from build123d import *

# Parameters (mm, degrees)
F0_W     = 0.6
F0_H     = 1.6
F1_DEPTH = 5
F3_DEPTH = 5
F4_W     = 5
F4_H     = 5
F5_DEPTH = 25


with BuildPart() as f1:
    # F0 (on Top) → F1 (new body)
    with BuildSketch(Plane.XY):
        with BuildLine():
            ThreePointArc((50, 7.5), (48.535534, 11.035534), (45, 12.5))
            Line((45, 12.5), (-45, 12.5))
            ThreePointArc((-45, 12.5), (-48.535534, 11.035534), (-50, 7.5))
            Line((-50, 7.5), (-50, -7.5))
            ThreePointArc((-50, -7.5), (-48.535534, -11.035534), (-45, -12.5))
            Line((-45, -12.5), (45, -12.5))
            ThreePointArc((45, -12.5), (48.535534, -11.035534), (50, -7.5))
            Line((50, -7.5), (50, 7.5))
        make_face()
        with Locations((-41, 0)):
            Rectangle(F0_W, F0_H, mode=Mode.SUBTRACT)
        with Locations((-35, 0)):
            Rectangle(F0_W, F0_H, mode=Mode.SUBTRACT)
        with Locations((15, 0)):
            Rectangle(F0_W, F0_H, mode=Mode.SUBTRACT)
        with Locations((21, 0)):
            Rectangle(F0_W, F0_H, mode=Mode.SUBTRACT)
    extrude(amount=F1_DEPTH)

    # F2 (on face) → F3 (join)
    with BuildSketch(Plane.XY.offset(5)):
        Polygon((25, -10.15), (27, -10.15), (27, 10.15), (45.5, 10.15), (45.5, -10.15), (47.5, -10.15), (47.5, 10.15), (47.5, 11.65), (25, 11.65), (25, 10.15), align=None)
    extrude(amount=F3_DEPTH)

    # F4 (on face) → F5 (cut)
    with BuildSketch(Plane(origin=(0, 11.65, 0), x_dir=(-1, 0, 0), z_dir=(0, 1, 0))):
        with Locations((-43, 7.5)):
            Rectangle(F4_W, F4_H)
    extrude(amount=-F5_DEPTH, mode=Mode.SUBTRACT)


solid = f1.part
Could you check a few things on this model? Use its own coordinates, in mm. A direction names the side the tool comes from. Give positions to 0.01 mm unless a question says otherwise; leave off trailing zeros. Loops run counter-clockwise (first coordinate to the right, second up) from the corner with the lowest first, then second, coordinate; pieces in that order, holes last. Notation, with made-up numbers: (-15.5, 21) -> (10.5, 21) arc R14 ccw to (10.5, 47) -> close; hole circle Ø6 at (-27, -17). An arc over 180 degrees is marked (long way). Answer as CSV lines item,"result". Start each with the question number.
(1) If we section it at A-A on y = -4.25: Write out the boundary of the cut face in (x, z).
(2) If we section it at B-B on x = -2: Write out the boundary of the cut face in (y, z), then the cut area to 3 significant figures.
(3) I'm going to push flat-ended pins straight in: pin 1 Ø2.5 at (y, z) = (5, 8.5) entering from +X; pin 2 Ø12 at (x, y) = (-33.5, 7.5) entering from +Z; pin 3 Ø2.5 at (y, z) = (-4.5, 6.5) entering from -X. Where does each tip first touch, or does it pass through?
(4) We'd pull the mould along Y, two halves only. Please class faces 4 (the flat face through (-41.3, 0, 2)), 5 (the flat face through (33, 11.65, 7)), 6 (the flat face through (45.5, 1, 7)): released by +Y, released by -Y, zero draft, split by the parting line, or undercut.
(5) I need wall thicknesses on probe 1 along X at (y, z) = (-6, 7.75); probe 2 along X at (y, z) = (10.5, 6.5); probe 3 along Z at (x, y) = (-17, 5). Which ranges of each line are inside material? Lowest first, please.
(6) Which directions (+Z, -Z, +X, -X, +Y, -Y) give clear straight access to the entire face, cutting with the end or side of a thin tool? Please do faces 1 (the flat face through (47.5, 1, 7)), 2 (the flat face through (15.3, 0, 2)), 3 (the flat face through (34, 10.15, 7)).
Computed:
1,outline,"(-50, 0) -> (50, 0) -> (50, 5) -> (47.5, 5) -> (47.5, 10) -> (45.5, 10) -> (45.5, 5) -> (27, 5) -> (27, 10) -> (25, 10) -> (25, 5) -> (-50, 5) -> close"
2,outline,"(-12.5, 0) -> (12.5, 0) -> (12.5, 5) -> (-12.5, 5) -> close"
2,area,"125 mm2"
3,pin 1,"stops at x = 47.5"
3,pin 2,"stops at z = 5"
3,pin 3,"stops at x = 25"
4,face 4,"undercut"
4,face 5,"released by +Y"
4,face 6,"zero draft"
5,probe 1,"x = 25 to 27, 45.5 to 47.5"
5,probe 2,"x = 25 to 40.5, 45.5 to 47.5"
5,probe 3,"z = 0 to 5"
6,face 1,"+Z, +X, +Y, -Y"
6,face 2,"+Z, -Z"
6,face 3,"+Z, -Y"
